Geometry check sheet. Reference: the model listing, model coordinates, mm. A direction names the side the tool comes from. Give positions to 0.01 mm unless a question says otherwise; leave off trailing zeros. Write each loop counter-clockwise with the first axis right and the second up, starting at its lowest first coordinate (ties: lowest second). Pieces come first, ordered by that corner, then holes. Notation, with made-up numbers: (24.25, 55.25) - (30.25, 55.25) arc R21 cw to (30.25, 63.25) - close; hole circle Ø2 at (23, 79.25). An arc over 180 degrees is marked (long way). Use a Markdown table: item, result.
```python
from build123d import *

# Parameters (mm, degrees)
SKETCH004_W       = 11.5
SKETCH004_H       = 1.25
PAD003_DEPTH      = 3.2
PAD005_DEPTH      = 40
PAD005_DEPTH_BACK = 1.6
THICKNESS001_T    = -1.6


with BuildPart() as pad003:
    # Sketch004 → Pad003 (new body)
    with BuildSketch(Plane.XZ.offset(46.2)):
        with BuildLine():
            Line((22.5, 29), (37.25, 29))
            ThreePointArc((38.25, 28), (37.957107, 28.707107), (37.25, 29))
            Line((38.25, 28), (38.25, 18))
            ThreePointArc((37.25, 17), (37.957107, 17.292893), (38.25, 18))
            Line((37.25, 17), (22.5, 17))
            ThreePointArc((21.5, 18), (21.792893, 17.292893), (22.5, 17))
            Line((21.5, 18), (21.5, 28))
            ThreePointArc((22.5, 29), (21.792893, 28.707107), (21.5, 28))
        make_face()
        with BuildLine():
            Line((-8.95, 29.8), (-3.75, 29.8))
            ThreePointArc((-2.75, 28.8), (-3.042893, 29.507107), (-3.75, 29.8))
            Line((-2.75, 28.8), (-2.75, 16.5))
            ThreePointArc((-3.75, 15.5), (-3.042893, 15.792893), (-2.75, 16.5))
            Line((-3.75, 15.5), (-8.95, 15.5))
            ThreePointArc((-9.95, 16.5), (-9.657107, 15.792893), (-8.95, 15.5))
            Line((-9.95, 16.5), (-9.95, 28.8))
            ThreePointArc((-8.95, 29.8), (-9.657107, 29.507107), (-9.95, 28.8))
        make_face()
        with BuildLine():
            Line((-37.25, 24.5), (-31.25, 24.5))
            ThreePointArc((-30.25, 23.5), (-30.542893, 24.207107), (-31.25, 24.5))
            Line((-30.25, 23.5), (-30.25, 18))
            ThreePointArc((-31.25, 17), (-30.542893, 17.292893), (-30.25, 18))
            Line((-31.25, 17), (-37.25, 17))
            ThreePointArc((-38.25, 18), (-37.957107, 17.292893), (-37.25, 17))
            Line((-38.25, 18), (-38.25, 23.5))
            ThreePointArc((-37.25, 24.5), (-37.957107, 24.207107), (-38.25, 23.5))
        make_face()
        with Locations((-20.25, 17.625)):
            Rectangle(SKETCH004_W, SKETCH004_H)
        Polygon((2.333401, 7), (2.333401, 11.006851), (3.391764, 12.4), (15.751917, 12.4), (16.833401, 10.855655), (16.833401, 7), align=None)
    extrude(amount=-PAD003_DEPTH)


with BuildPart() as cut001:
    # Sketch006 → Pad005 (new body, two sides)
    with BuildSketch(Plane.XY) as pad005_sk:
        with BuildLine():
            Line((-42.85, 44.6), (42.85, 44.6))
            ThreePointArc((47.85, 39.6), (46.385534, 43.135534), (42.85, 44.6))
            Line((47.85, 39.6), (47.85, -39.6))
            ThreePointArc((42.85, -44.6), (46.385534, -43.135534), (47.85, -39.6))
            Line((42.85, -44.6), (-42.85, -44.6))
            ThreePointArc((-47.85, -39.6), (-46.385534, -43.135534), (-42.85, -44.6))
            Line((-47.85, -39.6), (-47.85, 39.6))
            ThreePointArc((-42.85, 44.6), (-46.385534, 43.135534), (-47.85, 39.6))
        make_face()
    extrude(amount=PAD005_DEPTH)
    extrude(pad005_sk.sketch, amount=-PAD005_DEPTH_BACK)

    # Thickness001
    thickness001_openings = [cut001.faces().sort_by_distance(p)[0] for p in [
        (0, 0, 40),
    ]]
    offset(amount=THICKNESS001_T, openings=thickness001_openings)

    # Cut001: cut Pad003
    add(pad003.part, mode=Mode.SUBTRACT)


solid = cut001.part
```
1) Section check A-A on z = 20.5. Record the boundary of the cut face in (x, y).
Working result:
| item | result |
|---|---|
| outline | (-47.85, -39.6) arc R5 ccw to (-42.85, -44.6) - (-38.25, -44.6) - (-38.25, -43) - (-42.85, -43) arc R3.4 cw to (-46.25, -39.6) - (-46.25, 39.6) arc R3.4 cw to (-42.85, 43) - (42.85, 43) arc R3.4 cw to (46.25, 39.6) - (46.25, -39.6) arc R3.4 cw to (42.85, -43) - (38.25, -43) - (38.25, -44.6) - (42.85, -44.6) arc R5 ccw to (47.85, -39.6) - (47.85, 39.6) arc R5 ccw to (42.85, 44.6) - (-42.85, 44.6) arc R5 ccw to (-47.85, 39.6) - close; (-30.25, -44.6) - (-9.95, -44.6) - (-9.95, -43) - (-30.25, -43) - close; (-2.75, -44.6) - (21.5, -44.6) - (21.5, -43) - (-2.75, -43) - close |
2) Material ranges on L1, parallel to X at y = -7, z = 15; L2, parallel to Y at x = 19.5, z = 11.5; L3, parallel to Z at x = -7, y = 41, recorded low to high. Write a range as from..to.
Working result:
| item | result |
|---|---|
| L1 | x = -47.85..-46.25, 46.25..47.85 |
| L2 | y = -44.6..-43, 43..44.6 |
| L3 | z = -1.6..0 |
3) Set-up check for faces 4 (the cylindrical face through (-45.28, -41.98, 20.28)), 5 (the flat face through (21.5, 43.2, 40)): record each of +Z, -Z, +X, -X, +Y, -Y from which the full face is reachable in a straight line by a thin tool's end or side.
Working result:
| item | result |
|---|---|
| face 4 | +Z |
| face 5 | +Z, +X, -X, +Y, -Y |
4) Section check B-B on x = -19.5. Record the boundary of the cut face in (y, z).
Working result:
| item | result |
|---|---|
| outline | (-44.6, -1.6) - (44.6, -1.6) - (44.6, 40) - (43, 40) - (43, 0) - (-43, 0) - (-43, 17) - (-44.6, 17) - close; (-44.6, 18.25) - (-43, 18.25) - (-43, 40) - (-44.6, 40) - close |
5) Section check D-D on z = 35. Record the boundary of the cut face in (x, y), then the cut area to 3 significant figures.
Working result:
| item | result |
|---|---|
| outline | (-47.85, -39.6) arc R5 ccw to (-42.85, -44.6) - (42.85, -44.6) arc R5 ccw to (47.85, -39.6) - (47.85, 39.6) arc R5 ccw to (42.85, 44.6) - (-42.85, 44.6) arc R5 ccw to (-47.85, 39.6) - close; hole (-46.25, -39.6) arc R3.4 ccw to (-42.85, -43) - (42.85, -43) arc R3.4 ccw to (46.25, -39.6) - (46.25, 39.6) arc R3.4 ccw to (42.85, 43) - (-42.85, 43) arc R3.4 ccw to (-46.25, 39.6) - close |
| area | 570 mm² |
6) Depth check by flat-ended pin: P1, Ø0.6, axis at y = -44, z = 17.5, coming from the -X side; P2, Ø1.3, axis at y = -43.5, z = 22, coming from the -X side; P3, Ø1.5, axis at x = -21.5, y = -10.5, coming from the +Z side. Enter the tip coordinate at first touch or a pass-through.
Working result:
| item | result |
|---|---|
| P1 | stops at x = -45.71 |
| P2 | stops at x = -46.65 |
| P3 | stops at z = 0 |
7) Mould release check, pull along X, two halves, no side actions. Record for faces 1 (the flat face through (-1, 44.6, 19)), 2 (the flat face through (47.85, 1, 19)), 3 (the flat face through (1, 1, 0)): pulls with the +X half, pulls with the -X half, needs draft (parallel to the pull), parting line crosses it, or undercut.
Working result:
| item | result |
|---|---|
| face 1 | needs draft |
| face 2 | pulls with the +X half |
| face 3 | undercut |
8) Section check C-C on z = 26. Record the boundary of the cut face in (x, y), then the cut area to 3 significant figures.
Working result:
| item | result |
|---|---|
| outline | (-47.85, -39.6) arc R5 ccw to (-42.85, -44.6) - (-9.95, -44.6) - (-9.95, -43) - (-42.85, -43) arc R3.4 cw to (-46.25, -39.6) - (-46.25, 39.6) arc R3.4 cw to (-42.85, 43) - (42.85, 43) arc R3.4 cw to (46.25, 39.6) - (46.25, -39.6) arc R3.4 cw to (42.85, -43) - (38.25, -43) - (38.25, -44.6) - (42.85, -44.6) arc R5 ccw to (47.85, -39.6) - (47.85, 39.6) arc R5 ccw to (42.85, 44.6) - (-42.85, 44.6) arc R5 ccw to (-47.85, 39.6) - close; (-2.75, -44.6) - (21.5, -44.6) - (21.5, -43) - (-2.75, -43) - close |
| area | 532 mm² |
